```python
from build123d import *

# Parameters (mm, degrees)
SKETCH1_W                    = 75
SKETCH1_H                    = 130
BASE_FLANGE1_DEPTH           = 3.4163
EDGE_FLANGE1_STRIP_W         = 21.2852
EDGE_FLANGE1_STRIP_H         = 3.4163
EDGE_FLANGE1_STRIP_CUT_DEPTH = 130
EDGE_FLANGE1_DEPTH           = 130
SKETCH18_R                   = 37
SKETCH18_R_2                 = 4
CUT_EXTRUDE1_DEPTH           = 10
BREAK_CORNER1_DEPTH          = 3.4163
BREAK_CORNER2_START          = -3.4163
BREAK_CORNER2_DEPTH          = 3.4163
CUT_EXTRUDE2_DEPTH           = 10
EDGE_FLANGE2_DEPTH           = 30
EDGE_FLANGE3_DEPTH           = 22.7737
EDGE_FLANGE4_DEPTH           = 30
EDGE_FLANGE5_DEPTH           = 22.7737
BREAK_CORNER3_START          = 40.708137393
BREAK_CORNER3_OUTLINE_W      = 17
BREAK_CORNER3_OUTLINE_H      = 3.4163
BREAK_CORNER3_DEPTH          = 7.071067812
BREAK_CORNER4_START          = 3.76
BREAK_CORNER4_DEPTH          = 3.4163


# Read off the part's stored shape, not the designer's step: Break-Corner1, Break-Corner2, Break-Corner3, Break-Corner4
# Sheet-metal steps are written as plain solids
with BuildPart() as part:
    # Sketch1 → Base-Flange1 (new body)
    with BuildSketch(Plane(origin=(0, 0, 0), x_dir=(1, 0, 0), z_dir=(0, 1, 0))):
        with Locations((37.5, 65)):
            Rectangle(SKETCH1_W, SKETCH1_H)
    extrude(amount=-BASE_FLANGE1_DEPTH)

    # Edge-Flange1 strip (across the edge) → Edge-Flange1 strip cut (cut)
    with BuildSketch(Plane.XY.offset(-130)):
        with Locations((-3.4163, -1.70815)):
            Rectangle(EDGE_FLANGE1_STRIP_W, EDGE_FLANGE1_STRIP_H)
    extrude(amount=EDGE_FLANGE1_STRIP_CUT_DEPTH, mode=Mode.SUBTRACT)

    # Edge-Flange1 section (across the edge) → Edge-Flange1 (add)
    with BuildSketch(Plane.XY.offset(-130)):
        with BuildLine():
            Line((0, 3.81), (0, 96.5837))
            Line((0, 96.5837), (3.4163, 96.5837))
            Line((3.4163, 96.5837), (3.4163, 3.81))
            ThreePointArc((3.4163, 3.81), (4.532223164, 1.115923164), (7.2263, 0))
            Line((7.2263, 0), (7.2263, -3.4163))
            ThreePointArc((7.2263, -3.4163), (2.116534267, -1.299765733), (0, 3.81))
        make_face()
    extrude(amount=EDGE_FLANGE1_DEPTH)

    # Sketch18 → Cut-Extrude1 (cut)
    with BuildSketch(Plane.ZY):
        with Locations(Location((-65, 48.8287, 0), (0, 0, 270))):
            Circle(SKETCH18_R)
        with Locations(Location((-99.8, 83.6287, 0), (0, 0, 270))):
            Circle(SKETCH18_R_2)
        with Locations(Location((-30.2, 83.6287, 0), (0, 0, 270))):
            Circle(SKETCH18_R_2)
        with Locations(Location((-30.098341997, 13.953302375, 0), (0, 0, 270))):
            Circle(SKETCH18_R_2)
        with Locations(Location((-99.8, 14.0287, 0), (0, 0, 270))):
            Circle(SKETCH18_R_2)
    extrude(amount=-CUT_EXTRUDE1_DEPTH, mode=Mode.SUBTRACT)

    # Break-Corner1 outline → Break-Corner1 (cut)
    with BuildSketch(Plane.YZ):
        Polygon((96.5837, 0), (86.5837, 0), (96.5837, -10), align=None)
        Polygon((96.5837, -130), (96.5837, -120), (86.5837, -130), align=None)
    extrude(amount=BREAK_CORNER1_DEPTH, mode=Mode.SUBTRACT)

    # Break-Corner2 outline → Break-Corner2 (cut)
    with BuildSketch(Plane(origin=(0, 0, 0), x_dir=(1, 0, 0), z_dir=(0, 1, 0)).offset(BREAK_CORNER2_START)):
        Polygon((75, 0), (75, 10), (65, 0), align=None)
        Polygon((65, 130), (75, 120), (75, 130), align=None)
    extrude(amount=BREAK_CORNER2_DEPTH, mode=Mode.SUBTRACT)

    # Sketch19 → Cut-Extrude2 (cut)
    with BuildSketch(Plane(origin=(0, 0, 0), x_dir=(1, 0, 0), z_dir=(0, 1, 0))):
        with BuildLine():
            Line((67.28653865, 112), (14.54606135, 112))
            ThreePointArc((14.54606135, 112), (11.54606135, 115), (14.54606135, 118))
            Line((14.54606135, 118), (67.28653865, 118))
            ThreePointArc((67.28653865, 118), (70.28653865, 115), (67.28653865, 112))
        make_face()
        with BuildLine():
            Line((65.9163, 12), (15.9163, 12))
            ThreePointArc((15.9163, 12), (12.9163, 15), (15.9163, 18))
            Line((15.9163, 18), (65.9163, 18))
            ThreePointArc((65.9163, 18), (68.9163, 15), (65.9163, 12))
        make_face()
    extrude(amount=-CUT_EXTRUDE2_DEPTH, mode=Mode.SUBTRACT)

    # Edge-Flange2 section (across the edge) → Edge-Flange2 (add)
    with BuildSketch(Plane(origin=(10.9863, 0, 3.81), x_dir=(0, 0, -1), z_dir=(1, 0, 0))):
        with BuildLine():
            Line((-3.4163, 3.81), (-3.4163, 26.5837))
            Line((-3.4163, 26.5837), (0, 26.5837))
            Line((0, 26.5837), (0, 3.81))
            ThreePointArc((0, 3.81), (1.115923164, 1.115923164), (3.81, 0))
            Line((3.81, 0), (3.81, -3.4163))
            ThreePointArc((3.81, -3.4163), (-1.299765733, -1.299765733), (-3.4163, 3.81))
        make_face()
    extrude(amount=EDGE_FLANGE2_DEPTH)

    # Edge-Flange3 section (across the edge) → Edge-Flange3 (add)
    with BuildSketch(Plane(origin=(7.1763, 3.81, 3.81), x_dir=(1, 0, 0), z_dir=(0, 1, 0))):
        with BuildLine():
            Line((-3.4163, 3.81), (-3.4163, 16.5837))
            Line((-3.4163, 16.5837), (0, 16.5837))
            Line((0, 16.5837), (0, 3.81))
            ThreePointArc((0, 3.81), (1.115923164, 1.115923164), (3.81, 0))
            Line((3.81, 0), (3.81, -3.4163))
            ThreePointArc((3.81, -3.4163), (-1.299765733, -1.299765733), (-3.4163, 3.81))
        make_face()
    extrude(amount=EDGE_FLANGE3_DEPTH)

    # Edge-Flange4 section (across the edge) → Edge-Flange4 (add)
    with BuildSketch(Plane(origin=(40.9863, 0, -133.81), x_dir=(0, 0, 1), z_dir=(-1, 0, 0))):
        with BuildLine():
            Line((-3.4163, 3.81), (-3.4163, 26.5837))
            Line((-3.4163, 26.5837), (0, 26.5837))
            Line((0, 26.5837), (0, 3.81))
            ThreePointArc((0, 3.81), (1.115923164, 1.115923164), (3.81, 0))
            Line((3.81, 0), (3.81, -3.4163))
            ThreePointArc((3.81, -3.4163), (-1.299765733, -1.299765733), (-3.4163, 3.81))
        make_face()
    extrude(amount=EDGE_FLANGE4_DEPTH)

    # Edge-Flange5 section (across the edge) → Edge-Flange5 (add)
    with BuildSketch(Plane(origin=(7.1763, 26.5837, -133.81), x_dir=(1, 0, 0), z_dir=(0, -1, 0))):
        with BuildLine():
            Line((-3.4163, 3.81), (-3.4163, 16.5837))
            Line((-3.4163, 16.5837), (0, 16.5837))
            Line((0, 16.5837), (0, 3.81))
            ThreePointArc((0, 3.81), (1.115923164, 1.115923164), (3.81, 0))
            Line((3.81, 0), (3.81, -3.4163))
            ThreePointArc((3.81, -3.4163), (-1.299765733, -1.299765733), (-3.4163, 3.81))
        make_face()
    extrude(amount=EDGE_FLANGE5_DEPTH)

    # Break-Corner3 outline → Break-Corner3 (cut)
    with BuildSketch(Plane(origin=(0, 0, 0), x_dir=(0.7071067811865471, -0.707106781186548, 0), z_dir=(0.707106781186548, 0.707106781186547, 0)).offset(BREAK_CORNER3_START)):
        with Locations((10.5, -5.51815)):
            Rectangle(BREAK_CORNER3_OUTLINE_W, BREAK_CORNER3_OUTLINE_H)
        with Locations((10.5, 135.51815)):
            Rectangle(BREAK_CORNER3_OUTLINE_W, BREAK_CORNER3_OUTLINE_H)
    extrude(amount=BREAK_CORNER3_DEPTH, mode=Mode.SUBTRACT)

    # Break-Corner4 outline → Break-Corner4 (cut)
    with BuildSketch(Plane.YZ.offset(BREAK_CORNER4_START)):
        Polygon((3.81, -12.7737), (8.81, -12.7737), (3.81, -7.7737), align=None)
        Polygon((26.5837, -7.7737), (21.5837, -12.7737), (26.5837, -12.7737), align=None)
        Polygon((26.5837, -117.2263), (21.5837, -117.2263), (26.5837, -122.2263), align=None)
        Polygon((3.81, -122.2263), (8.81, -117.2263), (3.81, -117.2263), align=None)
    extrude(amount=BREAK_CORNER4_DEPTH, mode=Mode.SUBTRACT)


solid = part.part
```
Model file for the job. Use its own axes, mm. A direction names the side the tool comes from. Coordinates: 2 decimals unless noted, no trailing zeros. Loops run counter-clockwise (first coordinate to the right, second up) from the corner with the lowest first, then second, coordinate; pieces in that order, holes last. Notation, with made-up numbers: (40, 5.25) -> (77, 5.25) arc R7 ccw to (77, 15.25) -> close; hole circle Ø4 at (-30, 23.25). An arc over 180 degrees is marked (long way). Answer as a JSON object with one key per item and string values.
Q1. Cut at C-C (y = 62). List the corners of the cut face in (x, z), and give its area (3 significant figures).
Report:
{"outline": "(0, -130) -> (3.42, -130) -> (3.42, -99.58) -> (0, -99.58) -> close; (0, -30.42) -> (3.42, -30.42) -> (3.42, 0) -> (0, 0) -> close", "area": "208 mm2"}
Q2. Cut at B-B (z = -15). List the corners of the cut face in (x, y).
Report:
{"outline": "(0, 3.81) arc R7.23 ccw to (7.23, -3.42) -> (12.92, -3.42) -> (12.92, 0) -> (7.23, 0) arc R3.81 cw to (3.42, 3.81) -> (3.42, 96.58) -> (0, 96.58) -> close; (68.92, -3.42) -> (75, -3.42) -> (75, 0) -> (68.92, 0) -> close"}
Q3. Flat gauge pins, fed straight in: P1, Ø9, axis at y = 14.03, z = -99.8, coming from the +X side; P2, Ø1.7, axis at x = 57.5, y = -1.5, coming from the +Z side; P3, Ø1.7, axis at x = 34.5, y = -1.5, coming from the +Z side; P4, Ø12, axis at x = 33, y = 32.5, coming from the +Z side (3 decimals). Where does each tip first touch, or does it go through?
Report:
{"P1": "stops at x = 3.42", "P2": "stops at z = 0", "P3": "stops at z = 5.69", "P4": "passes through"}
Q4. Probe probe 1 along X at (y, z) = (16, -2); probe 2 along Y at (x, z) = (17.5, -48); probe 3 along Y at (x, z) = (2, -99). List the from-to ranges inside material, lowest first.
Report:
{"probe 1": "x = 0 to 3.42, 3.76 to 7.18", "probe 2": "y = -3.42 to 0", "probe 3": "y = -1.18 to 10.11, 17.95 to 34.23, 63.42 to 79.71, 87.55 to 96.58"}
Q5. Cut at D-D (x = 55). List the corners of the cut face in (y, z), and give its area (3 significant figures).
Report:
{"outline": "(-3.42, -130) -> (0, -130) -> (0, -118) -> (-3.42, -118) -> close; (-3.42, -112) -> (0, -112) -> (0, -18) -> (-3.42, -18) -> close; (-3.42, -12) -> (0, -12) -> (0, 0) -> (-3.42, 0) -> close", "area": "403 mm2"}
Q6. Cut at A-A (x = 26.5). List the corners of the cut face in (y, z).
Report:
{"outline": "(-3.42, -130) arc R7.23 ccw to (3.81, -137.23) -> (26.58, -137.23) -> (26.58, -133.81) -> (3.81, -133.81) arc R3.81 cw to (0, -130) -> (0, -118) -> (-3.42, -118) -> close; (-3.42, -112) -> (0, -112) -> (0, -18) -> (-3.42, -18) -> close; (-3.42, -12) -> (0, -12) -> (0, 0) arc R3.81 cw to (3.81, 3.81) -> (26.58, 3.81) -> (26.58, 7.23) -> (3.81, 7.23) arc R7.23 ccw to (-3.42, 0) -> close"}
Q7. 3-axis set-ups, long thin cutter, end or side, ignore diameter. For faces 1 (the flat face through (5.444, 6.275, -119.761)), 2 (the flat face through (15, 26.584, -134)), 3 (the flat face through (5.44, 24.12, -10.24)), 4 (the flat face through (7, 3.81, -130)), 5 (the flat face through (41, -2, -12)): which of +Z, -Z, +X, -X, +Y, -Y reach the whole face in a straight line?
Report:
{"face 1": "+X", "face 2": "+Z, -Z, +X, +Y", "face 3": "+X, +Y", "face 4": "+Z, -Z", "face 5": "+Y, -Y"}
Q8. Pull direction X, two halves, no side cores. Call faces 6 (the flat face through (3.76, 15, -6)), 7 (the cylindrical face through (8.3, 15.4, -132.7)), 8 (the flat face through (5, 15, -12.774)): released by +X, released by -X, zero draft, split by the parting line, or undercut.
Report:
{"face 6": "undercut", "face 7": "released by +X", "face 8": "zero draft"}
